Could you check a few things on this drawing? It's one solid part, dimensions in mm from its lowest x, y, z. A direction names the side the tool comes from. Give positions to 0.01 mm unless a question says otherwise; leave off trailing zeros. Write each loop counter-clockwise with the first axis right and the second up, starting at its lowest first coordinate (ties: lowest second). Pieces come first, ordered by that corner, then holes. Notation, with made-up numbers: (47.5, 27) -> (51.5, 27) arc R24 cw to (51.5, 51) -> close; hole circle Ø3 at (14.5, -22.5). An arc over 180 degrees is marked (long way). Use CSV: the item, a comma, the result in double quotes. Start each with the question number.
(1) Suppose I cut it at D-D on x = 29. List the corners of the cut face in (y, z) for me, plus the area to 3 significant figures.
(2) For pin 1 Ø1.5 at (x, z) = (30, 5) entering from +Y; pin 2 Ø0.8 at (y, z) = (8.5, 3.5) entering from +X; pin 3 Ø3.5 at (x, z) = (19, 5) entering from -Y, each with a flat end and sliding along its axis, tell me the tip position at first contact or that it passes through.
(3) Suppose I cut it at A-A on x = 12.5. List the corners of the cut face in (y, z) for me.
(4) Which directions (+Z, -Z, +X, -X, +Y, -Y) give clear straight access to the entire face, cutting with the end or side of a thin tool? Please do the marked faces 1, 2, 3 and 4.
(5) Suppose I cut it at B-B on z = 6. List the corners of the cut face in (x, y) for me.
(6) I need wall thicknesses on L1, parallel to X at y = 12, z = 1.75; L2, parallel to Y at x = 7.5, z = 9.5; L3, parallel to Y at x = 4.5, z = 11.5. Which ranges of each line are inside material? Lowest first, please. Write a range as [from, to].
(7) Suppose I cut it at C-C on y = 5.5. List the corners of the cut face in (x, z) for me.
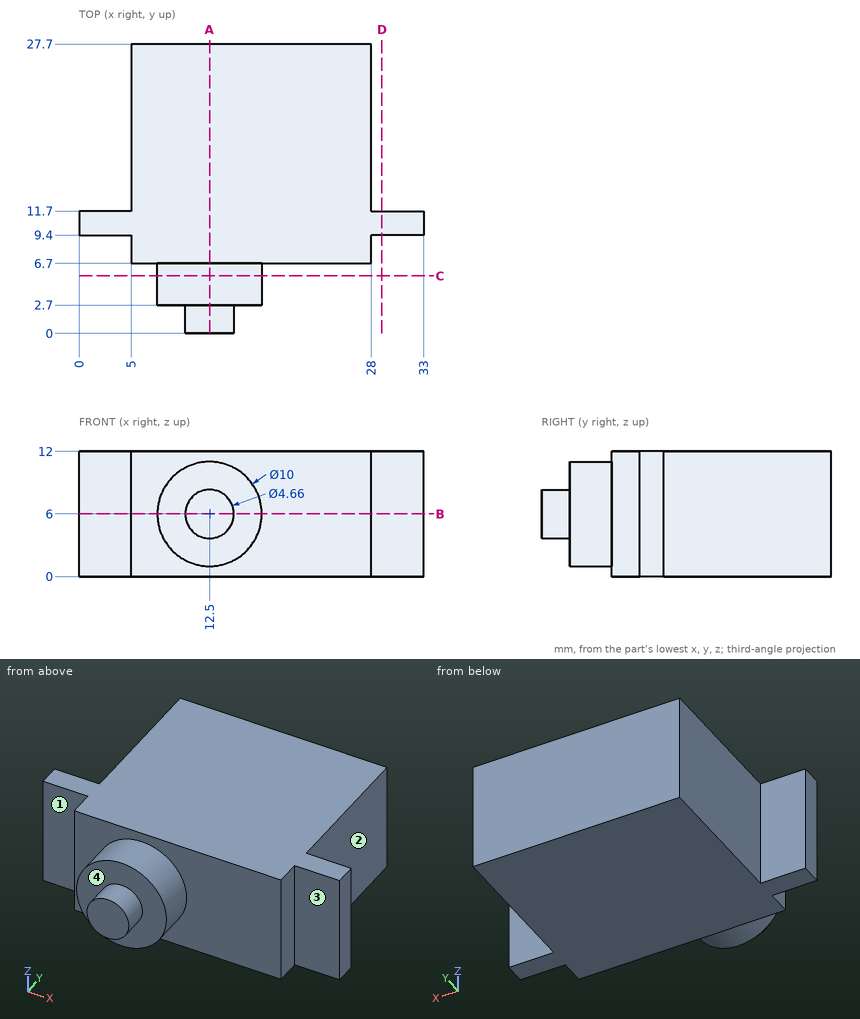
Geometry says:
1,outline,"(9.4, 0) -> (11.7, 0) -> (11.7, 12) -> (9.4, 12) -> close"
1,area,"27.6 mm²"
2,pin 1,"y = 11.7"
2,pin 2,"x = 28"
2,pin 3,"y = 2.7"
3,outline,"(0, 3.67) -> (2.7, 3.67) -> (2.7, 1) -> (6.7, 1) -> (6.7, 0) -> (27.7, 0) -> (27.7, 12) -> (6.7, 12) -> (6.7, 11) -> (2.7, 11) -> (2.7, 8.33) -> (0, 8.33) -> close"
4,face 1,"+Z, -Z, -X, -Y"
4,face 2,"+Z, -Z, +X, +Y"
4,face 3,"+Z, -Z, +X, -Y"
4,face 4,"-Y"
5,outline,"(0, 9.4) -> (5, 9.4) -> (5, 6.7) -> (7.5, 6.7) -> (7.5, 2.7) -> (10.17, 2.7) -> (10.17, 0) -> (14.83, 0) -> (14.83, 2.7) -> (17.5, 2.7) -> (17.5, 6.7) -> (28, 6.7) -> (28, 9.4) -> (33, 9.4) -> (33, 11.7) -> (28, 11.7) -> (28, 27.7) -> (5, 27.7) -> (5, 11.7) -> (0, 11.7) -> close"
6,L1,"[5, 28]"
6,L2,"[6.7, 27.7]"
6,L3,"[9.4, 11.7]"
7,outline,"circle Ø10 at (12.5, 6)"
